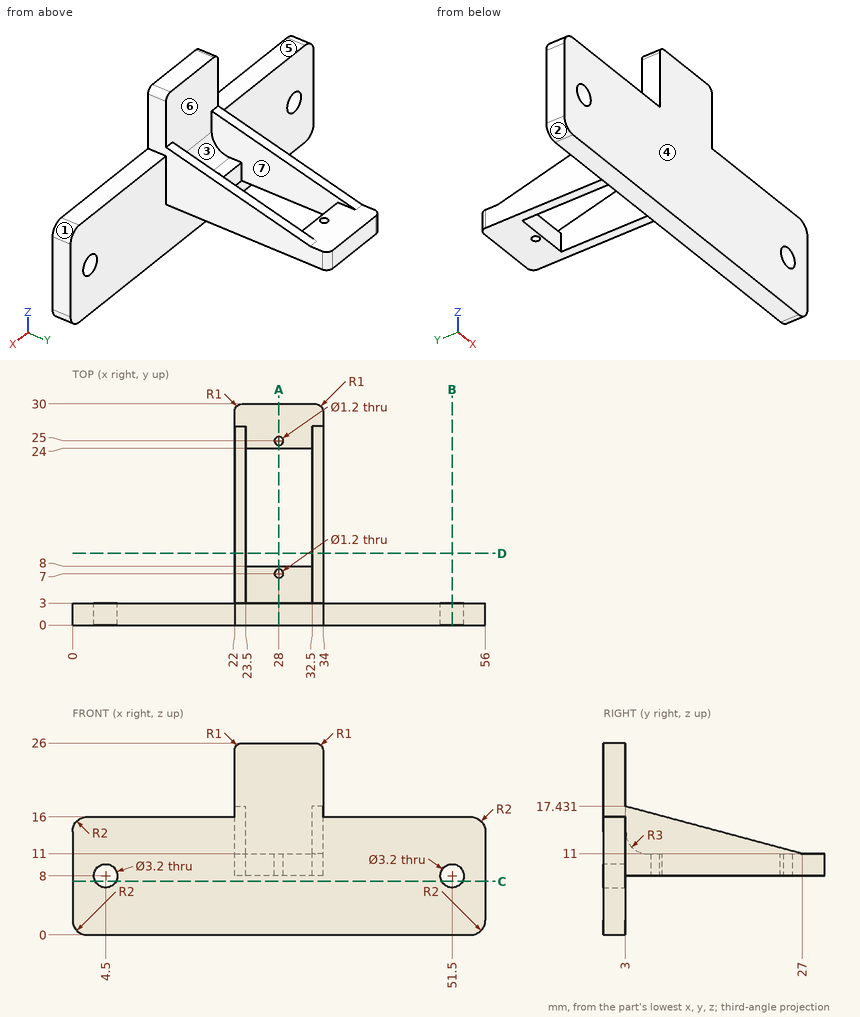
Answer from the drawing. Dimensions are ordinates in mm from the lowest x, y and z of the part. A direction names the side the tool comes from. Round coordinates to 2 decimals unless told otherwise and drop trailing zeros. Order: outer loops, then holes, each group sorted by start corner. A loop starts at its lowest first (then second) coordinate and runs counter-clockwise, first axis right, second up. Notation, with made-up numbers: (48, -6) - (72, -6) arc R27 ccw to (72, 10) - close; hole circle Ø5 at (-37, 37). An arc over 180 degrees is marked (long way). Put each result on its own line as item: value. Start each with the question number.
(1) Find section D-D (y = 9.75). Give the vertices of the cut face in (x, z), plus the area to 3 significant figures.
(2) For the marked faces 5, 6 and 7, determine the directions among +Z, -Z, +X, -X, +Y, -Y from which every point of the face is accessible in a straight line to the end or side of a thin tool.
(3) Straight lines are drawn through the part: probe 1 along X at (y, z) = (2.05, 8); probe 2 along Y at (x, z) = (28, 9.3); probe 3 along X at (y, z) = (5.5, 13.5). For each, find the intervals that lie inside material, in ascending order. Write a range as from..to.
(4) Find section B-B (x = 51.5). Give the vertices of the cut face in (y, z).
(5) Find section C-C (z = 7.25). Give the vertices of the cut face in (x, y).
(6) Determine the mould class of the marked faces 1, 2, 3 and 4 for opening direction X: released by +X, released by -X, zero draft, split by the parting line, or undercut.
(7) Given P1, Ø7.5, axis at y = 13, z = 11.5, coming from the +X side; P2, Ø4, axis at y = 5.5, z = 4, coming from the -X side; P3, Ø5, axis at x = 28.5, y = 25.5, coming from the +Z side; P4, Ø3.5, axis at x = 31, y = 16, coming from the -Z side, each flat-ended and moving along its own axis, determine where each tip first touches the part or whether it passes through.
(8) Find section A-A (x = 28). Give the vertices of the cut face in (y, z), plus the area to 3 significant figures.
Reply:
1. outline: (22, 8) - (23.5, 8) - (23.5, 15.62) - (22, 15.62) - close; (32.5, 8) - (34, 8) - (34, 15.62) - (32.5, 15.62) - close
1. area: 22.9 mm^2
2. face 5: +Z, -X, +Y, -Y
2. face 6: +Z, +Y
2. face 7: +Z
3. probe 1: 0..2.9, 6.1..49.9, 53.1..56
3. probe 2: 0..6.4, 7.6..8, 24..24.4, 25.6..30
3. probe 3: 22..23.5, 32.5..34
4. outline: (0, 0) - (3, 0) - (3, 6.4) - (0, 6.4) - close; (0, 9.6) - (3, 9.6) - (3, 16) - (0, 16) - close
5. outline: (0, 0) - (3.09, 0) - (3.09, 3) - (0, 3) - close; (5.91, 0) - (50.09, 0) - (50.09, 3) - (5.91, 3) - close; (52.91, 0) - (56, 0) - (56, 3) - (52.91, 3) - close
6. face 1: released by +X
6. face 2: released by -X
6. face 3: undercut
6. face 4: zero draft
7. P1: x = 34
7. P2: through
7. P3: z = 11
7. P4: z = 8
8. outline: (0, 0) - (3, 0) - (3, 8) - (6.4, 8) - (6.4, 11) - (6, 11) arc R3 cw to (3, 14) - (3, 26) - (0, 26) - close; (7.6, 8) - (8, 8) - (8, 11) - (7.6, 11) - close; (24, 8) - (24.4, 8) - (24.4, 11) - (24, 11) - close; (25.6, 8) - (30, 8) - (30, 11) - (25.6, 11) - close
8. area: 106 mm^2
